Drawing for the job (mm, zero at the part's lowest x, y, z). A direction names the side the tool comes from. Give positions to 0.01 mm unless a question says otherwise; leave off trailing zeros. Order: outer loops, then holes, each group sorted by start corner. A loop starts at its lowest first (then second) coordinate and runs counter-clockwise, first axis right, second up. Notation, with made-up numbers: (71, 83) - (94, 83) arc R30 cw to (94, 115) - close; hole circle Ø10 at (-15.75, 48.5). An arc over 180 degrees is marked (long way). One line per item, written item: value.
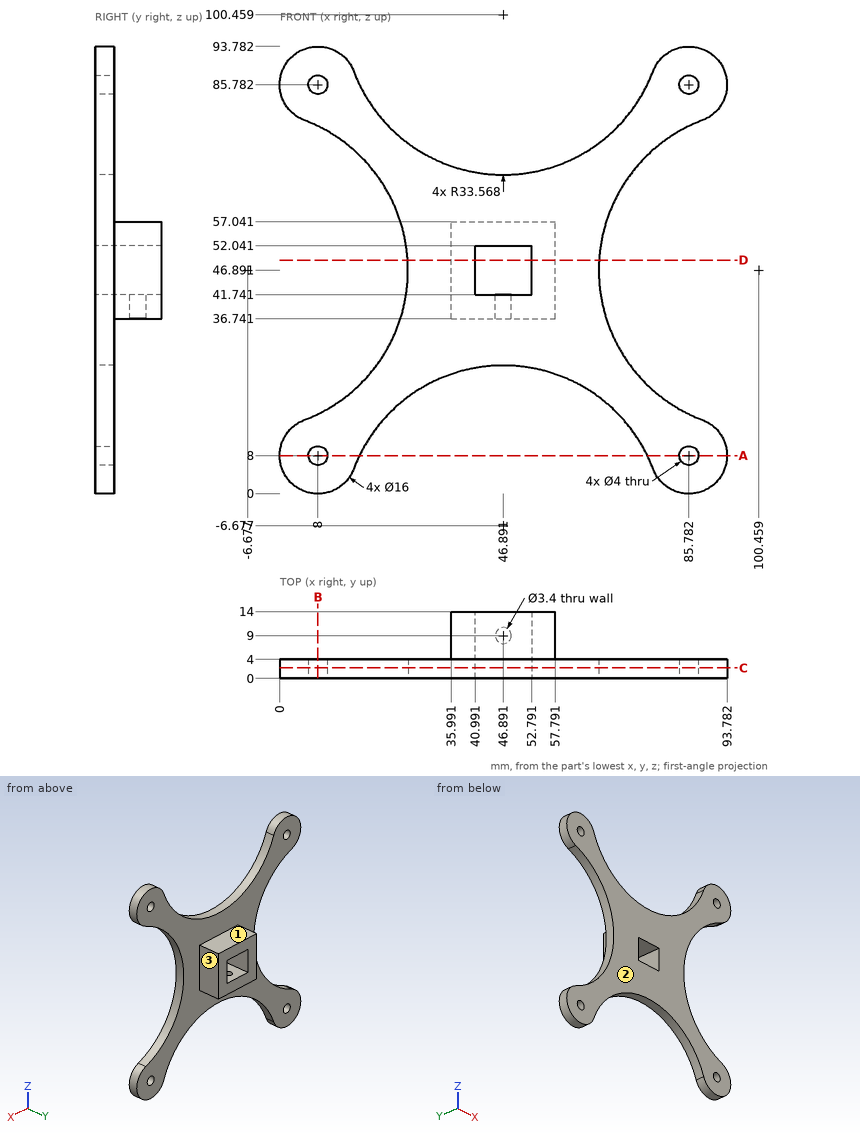
(1) Slice it at B-B, the plane x = 8. Give the cut face in (y, z).
Completed:
outline: (0, 0) - (4, 0) - (4, 6) - (0, 6) - close; (0, 10) - (4, 10) - (4, 16.7) - (0, 16.7) - close; (0, 77.08) - (4, 77.08) - (4, 83.78) - (0, 83.78) - close; (0, 87.78) - (4, 87.78) - (4, 93.78) - (0, 93.78) - close
(2) Drill centre lines: line 1 (X direction, y = 6.75, z = 45); line 2 (X direction, y = 1.05, z = 8); line 3 (Y direction, x = 61, z = 27). Where is each one in solid material? Low to high.
Completed:
line 1: 35.99 to 40.99, 52.79 to 57.79
line 2: 0 to 6, 10 to 16.7, 77.08 to 83.78, 87.78 to 93.78
line 3: 0 to 4
(3) Slice it at D-D, the plane z = 49. Give the cut face in (x, y) (1 decimal).
Completed:
outline: (26.8, 0) - (41, 0) - (41, 14) - (36, 14) - (36, 4) - (26.8, 4) - close; (52.8, 0) - (67, 0) - (67, 4) - (57.8, 4) - (57.8, 14) - (52.8, 14) - close
(4) Pin check, flat tips, straight feed: P1, Ø5, axis at x = 49, y = 9.5, coming from the +Z side; P2, Ø5, axis at y = 9, z = 51, coming from the -X side; P3, Ø8, axis at x = 52.5, y = 1.5, coming from the -Z side. Stop position of each tip, or through.
Completed:
P1: z = 57.04
P2: x = 35.99
P3: z = 25.49
(5) Slice it at A-A, the plane z = 8. Give the cut face in (x, y).
Completed:
outline: (0, 0) - (6, 0) - (6, 4) - (0, 4) - close; (10, 0) - (16.7, 0) - (16.7, 4) - (10, 4) - close; (77.08, 0) - (83.78, 0) - (83.78, 4) - (77.08, 4) - close; (87.78, 0) - (93.78, 0) - (93.78, 4) - (87.78, 4) - close
(6) Slice it at C-C, the plane y = 2.25. Give the cut face in (x, z) (1 decimal).
Completed:
outline: (5.2, 15.5) arc R8 ccw (long way) to (15.5, 5.2) arc R33.6 cw to (78.3, 5.2) arc R8 ccw (long way) to (88.6, 15.5) arc R33.6 cw to (88.6, 78.3) arc R8 ccw (long way) to (78.3, 88.6) arc R33.6 cw to (15.5, 88.6) arc R8 ccw (long way) to (5.2, 78.3) arc R33.6 cw to start; hole circle Ø4 at (8, 8); hole circle Ø4 at (8, 85.8); hole (41, 41.7) - (52.8, 41.7) - (52.8, 52) - (41, 52) - close; hole circle Ø4 at (85.8, 8); hole circle Ø4 at (85.8, 85.8)
(7) 3-axis set-ups, long thin cutter, end or side, ignore diameter. For the marked faces 1, 2 and 3: which of +Z, -Z, +X, -X, +Y, -Y reach the whole face in a straight line?
Completed:
face 1: +Z, +X, -X, +Y
face 2: +Z, -Z, +X, -X, -Y
face 3: +Z, -Z, +X, +Y
